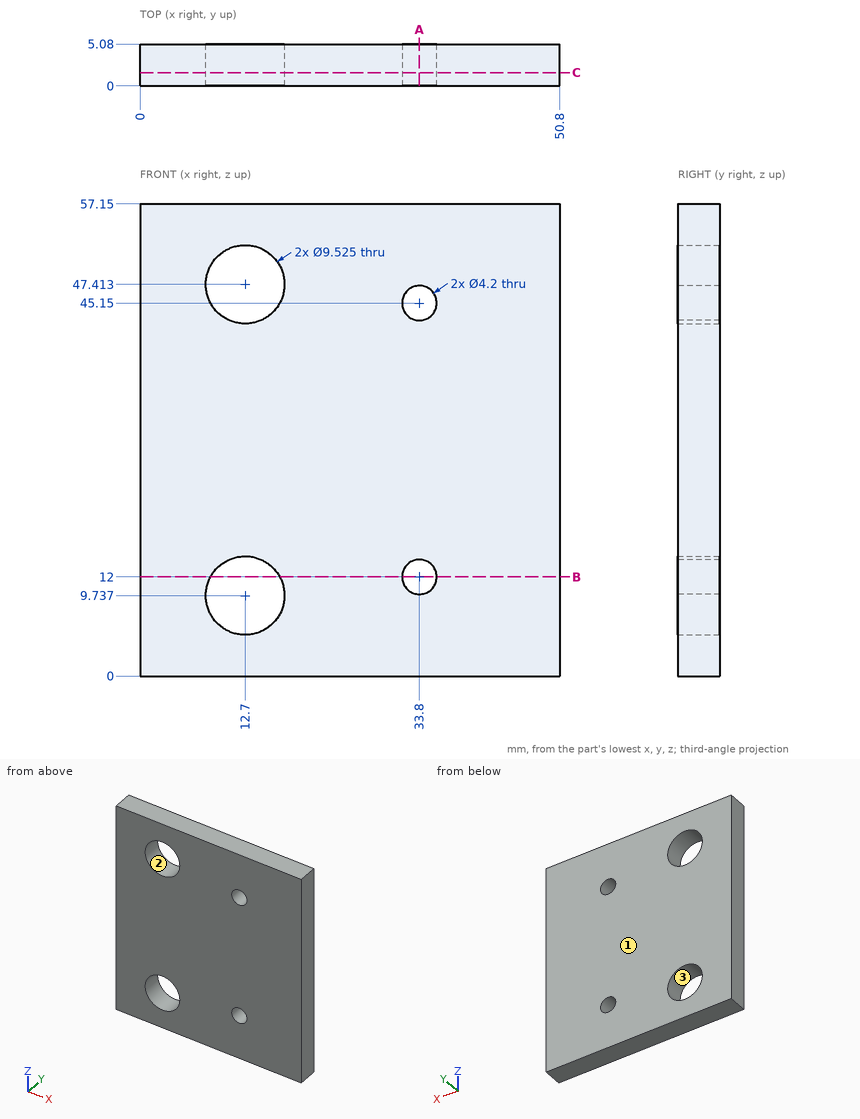
Input: dimensioned drawing with shaded views. Units: mm. Origin: part minimum x, y, z. Give positions to 0.01 mm unless a question says otherwise; leave off trailing zeros. Loops run counter-clockwise (first coordinate to the right, second up) from the corner with the lowest first, then second, coordinate; pieces in that order, holes last. Notation, with made-up numbers: M -10,30 L 40,30 A28 cw 40,58 Z; hole C -35.75,89.25 d5. An arc over 180 degrees is marked long. Put each result on its own line as item: value. Start each with the question number.
1) Cut plane A-A (x = 33.8). Output: boundary loops of the cut face in (y, z), then the cut area to 3 significant figures.
2) Pull-direction query (X, two-part tool) for the marked faces 1, 2 and 3; classes: pulls with the +X half, pulls with the -X half, needs draft (parallel to the pull), parting line crosses it, or undercut.
3) Cut plane B-B (z = 12). Output: boundary loops of the cut face in (x, y), then the cut area to 3 significant figures.
4) Cut plane C-C (y = 1.6). Give the number of separate pieces and of enclosed holes in the cut face, then the cut area to 3 significant figures.
5) Ray query, line 1 along X through (y, z) = (1.4, 9.5); line 2 along X through (y, z) = (4.8, 5.5) (1 decimal); line 3 along Z through (x, y) = (12, 2.25). Return the intervals inside material, ascending.
Verdict:
1. outline: M 0,0 L 5.08,0 L 5.08,9.9 L 0,9.9 Z; M 0,14.1 L 5.08,14.1 L 5.08,43.05 L 0,43.05 Z; M 0,47.25 L 5.08,47.25 L 5.08,57.15 L 0,57.15 Z
1. area: 248 mm2
2. face 1: needs draft
2. face 2: undercut
2. face 3: undercut
3. outline: M 0,0 L 8.51,0 L 8.51,5.08 L 0,5.08 Z; M 16.89,0 L 31.7,0 L 31.7,5.08 L 16.89,5.08 Z; M 35.9,0 L 50.8,0 L 50.8,5.08 L 35.9,5.08 Z
3. area: 194 mm2
4. separate pieces: 1
4. enclosed holes: 4
4. area: 2,730 mm2
5. line 1: 0 to 7.94, 17.46 to 50.8
5. line 2: 0 to 10.5, 14.9 to 50.8
5. line 3: 0 to 5.03, 14.45 to 42.7, 52.12 to 57.15
